Could you check a few things on this model? Use its own coordinates, in mm. A direction names the side the tool comes from. Give positions to 0.01 mm unless a question says otherwise; leave off trailing zeros. Order: outer loops, then holes, each group sorted by start corner. A loop starts at its lowest first (then second) coordinate and runs counter-clockwise, first axis right, second up. Notation, with made-up numbers: (65, 42) -> (93, 42) arc R15 cw to (93, 59) -> close; hole circle Ø4 at (-22.5, -33). An arc over 180 degrees is marked (long way). One line per item, written item: value.
```python
from build123d import *

# Parameters (mm, degrees)
SKETCH_1_R          = 4
EXTRUDE_1_DEPTH     = 91.56
SKETCH_2_R          = 20
EXTRUDE_2_DEPTH     = 14
SKETCH_3_R          = 15
EXTRUDE_3_DEPTH     = 12
SKETCH_4_R          = 20
SKETCH_4_R_2        = 17
CUT_EXTRUDE_1_DEPTH = 13
SKETCH_5_R          = 20
EXTRUDE_4_DEPTH     = 1


with BuildPart() as part:
    # 草图1 → 凸台-拉伸1 (new body)
    with BuildSketch(Plane.XY):
        Circle(SKETCH_1_R)
    extrude(amount=EXTRUDE_1_DEPTH)

    # 草图2 → 凸台-拉伸2 (add)
    with BuildSketch(Plane.XY.offset(91.56)):
        Circle(SKETCH_2_R)
    extrude(amount=EXTRUDE_2_DEPTH)

    # 草图3 → 凸台-拉伸3 (add)
    with BuildSketch(Plane.XY.offset(105.56)):
        Circle(SKETCH_3_R)
    extrude(amount=EXTRUDE_3_DEPTH)

    # 草图4 → 切除-拉伸1 (cut)
    with BuildSketch(Plane(origin=(0, 0, 91.56), x_dir=(-1, 0, 0), z_dir=(0, 0, -1))):
        Circle(SKETCH_4_R)
        Circle(SKETCH_4_R_2, mode=Mode.SUBTRACT)
    extrude(amount=-CUT_EXTRUDE_1_DEPTH, mode=Mode.SUBTRACT)

    # 草图5 → 凸台-拉伸4 (add)
    with BuildSketch(Plane(origin=(0, 0, 91.56), x_dir=(-1, 0, 0), z_dir=(0, 0, -1))):
        Circle(SKETCH_5_R)
    extrude(amount=-EXTRUDE_4_DEPTH)


solid = part.part
```
1) Suppose I cut it at A-A, the plane x = 0. Write out the boundary of the cut face in (y, z).
Answer below:
outline: (-20, 91.56) -> (-4, 91.56) -> (-4, 0) -> (4, 0) -> (4, 91.56) -> (20, 91.56) -> (20, 92.56) -> (17, 92.56) -> (17, 104.56) -> (20, 104.56) -> (20, 105.56) -> (15, 105.56) -> (15, 117.56) -> (-15, 117.56) -> (-15, 105.56) -> (-20, 105.56) -> (-20, 104.56) -> (-17, 104.56) -> (-17, 92.56) -> (-20, 92.56) -> close
2) If I drill on line 1 along Z through (x, y) = (16, 7); line 2 along Z through (x, y) = (-7.5, -8); line 3 along Z through (x, y) = (1, 15.5), over which ranges is the centre line in solid material (lowest first)?
Answer below:
line 1: z = 91.56 to 92.56, 104.56 to 105.56
line 2: z = 91.56 to 117.56
line 3: z = 91.56 to 105.56
3) For P1, Ø10, axis at x = -2.5, y = 15, coming from the -Z side; P2, Ø6, axis at y = 6.5, z = 86, coming from the +X side; P3, Ø8, axis at x = -3.5, z = 13, coming from the -Y side, each with a flat end and sliding along its axis, tell me the tip position at first contact or that it passes through.
Answer below:
P1: stops at z = 91.56
P2: stops at x = 1.94
P3: stops at y = -4
4) For faces 5 (the flat face through (9, -15, 92.56)), 6 (the cylindrical face through (-14.985, 0.66, 111.476)), 7 (the cylindrical face through (-4.336, -19.524, 105.053)), 8 (the cylindrical face through (-0.867, -3.905, 45.139)), which set-ups out of +Z, -Z, +X, -X, +Y, -Y let a thin tool reach every point of the face, with its end or its side?
Answer below:
face 5: none
face 6: +Z
face 7: +Z, -Z
face 8: -Z
5) Suppose I cut it at C-C, the plane z = 24.5. Write out the boundary of the cut face in (x, y), then the cut area to 3 significant figures.
Answer below:
outline: circle Ø8 at (0, 0)
area: 50.3 mm2
6) We'd pull the mould along Z, two halves only. Please class faces 1 (the cylindrical face through (4.336, -19.524, 92.053)), 2 (the flat face through (0, 0, 117.56)), 3 (the flat face through (0, 0, 0)), 4 (the flat face through (9, -15, 104.56)): +Z half, -Z half, draft (parallel to the pull), parting line (faces both ways), or undercut.
Answer below:
face 1: draft
face 2: +Z half
face 3: -Z half
face 4: undercut
7) Suppose I cut it at D-D, the plane x = 11. Write out the boundary of the cut face in (y, z), then the cut area to 3 significant figures.
Answer below:
outline: (-16.7, 91.56) -> (16.7, 91.56) -> (16.7, 92.56) -> (12.96, 92.56) -> (12.96, 104.56) -> (16.7, 104.56) -> (16.7, 105.56) -> (10.2, 105.56) -> (10.2, 117.56) -> (-10.2, 117.56) -> (-10.2, 105.56) -> (-16.7, 105.56) -> (-16.7, 104.56) -> (-12.96, 104.56) -> (-12.96, 92.56) -> (-16.7, 92.56) -> close
area: 623 mm2
